from build123d import *

# Parameters (mm, degrees)
ESQUISSE1_W                               = 16
ESQUISSE1_H                               = 8
BOSS_EXTRU_1_DEPTH                        = 6
TROU_POUR_TARAUDAGE_POUR_TROU_TARAUD_M3_D = 2.5
ESQUISSE4_R                               = 1.6
ENL_V_MAT_EXTRU_1_DEPTH                   = 6


with BuildPart() as part:
    # Esquisse1 → Boss.-Extru.1 (new body)
    with BuildSketch(Plane.XY):
        with Locations((1.433962264, 4)):
            Rectangle(ESQUISSE1_W, ESQUISSE1_H)
    extrude(amount=BOSS_EXTRU_1_DEPTH)

    # Trou pour taraudage pour trou taraudé M31 (through all)
    with Locations(Plane(origin=(0, 8, 0), x_dir=(1, 0, 0), z_dir=(0, 1, 0))):
        with Locations((-2.566037736, -3), (5.433962264, -3)):
            Hole(TROU_POUR_TARAUDAGE_POUR_TROU_TARAUD_M3_D / 2)

    # Esquisse4 → Enlèv. mat.-Extru.1 (cut)
    with BuildSketch(Plane.XY.offset(6)):
        with Locations((1.433962264, 4)):
            Circle(ESQUISSE4_R)
    extrude(amount=-ENL_V_MAT_EXTRU_1_DEPTH, mode=Mode.SUBTRACT)


solid = part.part
Work out the finished part from the listing and answer in its coordinate system (mm). Give positions to 0.01 mm unless a question says otherwise; leave off trailing zeros. Order: outer loops, then holes, each group sorted by start corner. A loop starts at its lowest first (then second) coordinate and runs counter-clockwise, first axis right, second up. Notation, with made-up numbers: M 10.25,50 L 21.25,50 A32 cw 21.25,81 Z; hole C -30,-35 d7. An arc over 180 degrees is marked long. Return JSON: item names as keys, results as strings.
Q1. Find section C-C, the plane x = -3.5. Write down the section's boundary in (y, z), and give its area (3 significant figures).
Answer below:
{"outline": "M 0,0 L 8,0 L 8,2.17 L 0,2.17 Z; M 0,3.83 L 8,3.83 L 8,6 L 0,6 Z", "area": "34.7 mm^2"}
Q2. The mould has two halves that part along Y. Classify faces 1 (the face through (1, 2, 6)), 2 (the face through (1.087, 2.438, 3.042)), 3 (the face through (1, 8, 3)): pulls with the +Y half, pulls with the -Y half, needs draft (parallel to the pull), parting line crosses it, or undercut.
Answer below:
{"face 1": "needs draft", "face 2": "undercut", "face 3": "pulls with the +Y half"}
Q3. Find section A-A, the plane y = 4. Write down the section's boundary in (x, z).
Answer below:
{"outline": "M -6.57,0 L -0.17,0 L -0.17,6 L -6.57,6 Z; M 3.03,0 L 9.43,0 L 9.43,6 L 3.03,6 Z; hole C -2.57,3 d2.5; hole C 5.43,3 d2.5"}
Q4. Find section D-D, the plane z = 4.55. Write down the section's boundary in (x, y).
Answer below:
{"outline": "M -6.57,0 L 9.43,0 L 9.43,8 L -6.57,8 Z; hole C 1.43,4 d3.2"}
Q5. This flat-tipped pin is pushed along its axis until it touches: pin 1 (1.9 mm diameter, centred on x = 1.43, y = 4, fed in from -Z). Where does it stop, or does it pass through?
Answer below:
{"pin 1": "passes through"}
Q6. Find the intervals of material crossed by line 1 along Z through (x, y) = (5.5, 0.75); line 2 along X through (y, z) = (2, 2.8); line 3 along X through (y, z) = (4.5, 4), in increasing order. Write a range as [from, to].
Answer below:
{"line 1": "z = [0, 1.75], [4.25, 6]", "line 2": "x = [-6.57, -3.8], [-1.33, 4.2], [6.67, 9.43]", "line 3": "x = [-6.57, -3.32], [-1.82, -0.09], [2.95, 4.68], [6.18, 9.43]"}
Q7. Find section B-B, the plane z = 3. Write down the section's boundary in (x, y), and give its area (3 significant figures).
Answer below:
{"outline": "M -6.57,0 L -3.82,0 L -3.82,8 L -6.57,8 Z; M -1.32,0 L 4.18,0 L 4.18,8 L -1.32,8 Z; M 6.68,0 L 9.43,0 L 9.43,8 L 6.68,8 Z; hole C 1.43,4 d3.2", "area": "80.0 mm^2"}
